```python
from build123d import *

# Parameters (mm, degrees)
SKETCH_1_W           = 80
SKETCH_1_H           = 60
SKETCH_1_R           = 2.1
SKETCH_1_W_2         = 40
SKETCH_1_H_2         = 24
EXTRUDE_1_DEPTH      = 10
CUT_EXTRUDE_1_DEPTH  = 80
SKETCH_5_W           = 5
SKETCH_5_H           = 3
CUT_EXTRUDE_2_DEPTH  = 80
SKETCH_7_W           = 56
SKETCH_7_H           = 24
CUT_EXTRUDE_3_DEPTH  = 1
SKETCH_8_W           = 40
SKETCH_8_H           = 40
EXTRUDE_2_DEPTH      = 3
SKETCH_9_W           = 10
SKETCH_9_H           = 60
CUT_EXTRUDE_4_DEPTH  = 10
CUT_EXTRUDE_11_DEPTH = 28
CUT_EXTRUDE_12_DEPTH = 41
SKETCH_24_W          = 10
SKETCH_24_H          = 10
EXTRUDE_3_DEPTH      = 70
SKETCH_25_W          = 12
SKETCH_25_H          = 6
CUT_EXTRUDE_13_DEPTH = 9
SKETCH_26_R          = 2
CUT_EXTRUDE_14_DEPTH = 8
CUT_EXTRUDE_15_REACH = 65.828
EXTRUDE_START        = -28
SKETCH_28_W          = 70
SKETCH_28_H          = 2
EXTRUDE_4_DEPTH      = 28
CUT_EXTRUDE_START    = -70
SKETCH_29_W          = 14
SKETCH_29_H          = 2
CUT_EXTRUDE_16_DEPTH = 70


with BuildPart() as part:
    # 草圖1 → 填料-伸長1 (new body)
    with BuildSketch(Plane(origin=(0, 0, 0), x_dir=(1, 0, 0), z_dir=(0, 1, 0))):
        Rectangle(SKETCH_1_W, SKETCH_1_H)
        with Locations(Location((-34.5, -5, 0), (0, 0, 270))):
            Circle(SKETCH_1_R, mode=Mode.SUBTRACT)
        with Locations(Location((-34.5, 5, 0), (0, 0, 270))):
            Circle(SKETCH_1_R, mode=Mode.SUBTRACT)
        with Locations(Location((15, -5, 0), (0, 0, 270))):
            Circle(SKETCH_1_R, mode=Mode.SUBTRACT)
        with Locations(Location((15, 5, 0), (0, 0, 270))):
            Circle(SKETCH_1_R, mode=Mode.SUBTRACT)
        with Locations((-10, 0)):
            Rectangle(SKETCH_1_W_2, SKETCH_1_H_2, mode=Mode.SUBTRACT)
    extrude(amount=EXTRUDE_1_DEPTH)

    # 草圖4 → 除料-伸長1 (cut)
    with BuildSketch(Plane(origin=(40, 0, 0), x_dir=(0, 0, -1), z_dir=(1, 0, 0))):
        Polygon((17, 10), (17, 8), (15, 8), (15, 3), (25, 3), (25, 8), (23, 8), (23, 10), align=None)
    extrude(amount=-CUT_EXTRUDE_1_DEPTH, mode=Mode.SUBTRACT)

    # 草圖5 → 除料-伸長2 (cut)
    with BuildSketch(Plane(origin=(0, 10, 0), x_dir=(1, 0, 0), z_dir=(0, 1, 0))):
        with Locations((12.5, 0)):
            Rectangle(SKETCH_5_W, SKETCH_5_H)
        with Locations((-32.5, 0)):
            Rectangle(SKETCH_5_W, SKETCH_5_H)
    extrude(amount=-CUT_EXTRUDE_2_DEPTH, mode=Mode.SUBTRACT)

    # 草圖7 → 除料-伸長3 (cut)
    with BuildSketch(Plane(origin=(0, 10, 0), x_dir=(1, 0, 0), z_dir=(0, 1, 0))):
        with Locations((-9.7, 0)):
            Rectangle(SKETCH_7_W, SKETCH_7_H)
    extrude(amount=-CUT_EXTRUDE_3_DEPTH, mode=Mode.SUBTRACT)

    # 草圖8 → 填料-伸長2 (add)
    with BuildSketch(Plane.ZY.offset(40)):
        with Locations((10, 5)):
            Rectangle(SKETCH_8_W, SKETCH_8_H)
    extrude(amount=EXTRUDE_2_DEPTH)

    # 草圖9 → 除料-伸長4 (cut)
    with BuildSketch(Plane(origin=(0, 10, 0), x_dir=(1, 0, 0), z_dir=(0, 1, 0))):
        with Locations((35, 0)):
            Rectangle(SKETCH_9_W, SKETCH_9_H)
    extrude(amount=-CUT_EXTRUDE_4_DEPTH, mode=Mode.SUBTRACT)

    # 草圖22 → 除料-伸長11 (cut)
    with BuildSketch(Plane(origin=(0, 10, 0), x_dir=(1, 0, 0), z_dir=(0, 1, 0))):
        Polygon((-43, -25), (-43, -30), (-38, -30), align=None)
    extrude(amount=-CUT_EXTRUDE_11_DEPTH, mode=Mode.SUBTRACT)

    # 草圖23 → 除料-伸長12 (cut)
    with BuildSketch(Plane(origin=(0, 25, 0), x_dir=(1, 0, 0), z_dir=(0, 1, 0))):
        Polygon((-43, -30), (-38, -30), (-43, -25), align=None)
    extrude(amount=-CUT_EXTRUDE_12_DEPTH, mode=Mode.SUBTRACT)

    # 草圖24 → 填料-伸長3 (add)
    with BuildSketch(Plane.ZY.offset(40)):
        with Locations((-35, 5)):
            Rectangle(SKETCH_24_W, SKETCH_24_H)
    extrude(amount=-EXTRUDE_3_DEPTH)

    # 草圖25 → 除料-伸長13 (cut)
    with BuildSketch(Plane(origin=(0, 10, 0), x_dir=(1, 0, 0), z_dir=(0, 1, 0))):
        with Locations((-12, 32)):
            Rectangle(SKETCH_25_W, SKETCH_25_H)
        with Locations((20, 32)):
            Rectangle(SKETCH_25_W, SKETCH_25_H)
    extrude(amount=-CUT_EXTRUDE_13_DEPTH, mode=Mode.SUBTRACT)

    # 草圖26 → 除料-伸長14 (cut)
    with BuildSketch(Plane(origin=(0, 0, -40), x_dir=(-1, 0, 0), z_dir=(0, 0, -1))):
        with Locations((-20, 4.723394197)):
            Circle(SKETCH_26_R)
        with Locations((12, 4.723394197)):
            Circle(SKETCH_26_R)
    extrude(amount=-CUT_EXTRUDE_14_DEPTH, mode=Mode.SUBTRACT)

    # 草圖27 → 除料-伸長15 (cut, up to next)
    with BuildSketch(Plane(origin=(0, 10, 0), x_dir=(1, 0, 0), z_dir=(0, 1, 0)), mode=Mode.PRIVATE) as cut_extrude_15_sk1:
        Polygon((30, -10), (20, -30), (30, -30), align=None)
    cut_extrude_15_tool1 = extrude(cut_extrude_15_sk1.sketch, amount=-CUT_EXTRUDE_15_REACH, mode=Mode.PRIVATE) & part.part
    add(cut_extrude_15_tool1.solids().sort_by_distance((26.666667, 10, 23.333333))[0], mode=Mode.SUBTRACT)

    # 草圖28 → 填料-伸長4 (add)
    with BuildSketch(Plane(origin=(0, 0, -40), x_dir=(-1, 0, 0), z_dir=(0, 0, -1)).offset(EXTRUDE_START)):
        with Locations((5, -1)):
            Rectangle(SKETCH_28_W, SKETCH_28_H)
    extrude(amount=EXTRUDE_4_DEPTH)

    # 草圖29 → 除料-伸長16 (cut)
    with BuildSketch(Plane(origin=(30, 0, 0), x_dir=(0, 0, -1), z_dir=(1, 0, 0)).offset(CUT_EXTRUDE_START)):
        with Locations((33, -1)):
            Rectangle(SKETCH_29_W, SKETCH_29_H)
    extrude(amount=CUT_EXTRUDE_16_DEPTH, mode=Mode.SUBTRACT)


solid = part.part
```
CAD build for the part. Positions are in the model's coordinates, mm. A direction names the side the tool comes from. Give positions to 0.01 mm unless a question says otherwise; leave off trailing zeros. Write each loop counter-clockwise with the first axis right and the second up, starting at its lowest first coordinate (ties: lowest second). Pieces come first, ordered by that corner, then holes. Notation, with made-up numbers: M 42.25,-39 L 68.25,-39 A11 cw 68.25,-34 Z; hole C 15,70.25 d6. An arc over 180 degrees is marked long. Return JSON: item names as keys, results as strings. Group by question number.
(1) Band-saw the part on C-C (x = -19.5). Give the cut face in (y, z), and give its area (3 significant figures).
(2) Mould opens along Z. For faces 1 (the face through (25, 5, 20)), 2 (the face through (21, 7, -35)), 3 (the face through (-5, -2, -19)), 4 (the face through (-5, -1, -26)) say: pulls with the +Z half, pulls with the -Z half, needs draft (parallel to the pull), parting line crosses it, or undercut.
(3) Drill centre lines: L1, parallel to Z at x = -34.5, y = 5.75; L2, parallel to Z at x = -10.5, y = 6; L3, parallel to Z at x = 5.5, y = 2.5. Where is each one in solid material? Low to high. Write a range as [from, to].
(4) Band-saw the part on A-A (x = -12). Give the cut face in (y, z).
(5) 3-axis set-ups, long thin cutter, end or side, ignore diameter. For faces 5 (the face through (-40, 2.6, -24.8)), 6 (the face through (20, 1, -32)), 7 (the face through (-10.53, 6.08, -37.53)), 8 (the face through (-5, 6, -15)), 9 (the face through (-33, 5, 1.5)): which of +Z, -Z, +X, -X, +Y, -Y reach the whole face in a straight line?
(6) Band-saw the part on D-D (z = 19). Give the cut face in (x, y).
(7) Band-saw the part on B-B (z = 5). Give the cut face in (x, y).
(8) Flat gauge pins, fed straight in: pin 1 Ø4 at (y, z) = (18, 1.5) entering from +X; pin 2 Ø7 at (x, z) = (6.5, -22) entering from -Y; pin 3 Ø3 at (x, z) = (-14, -28) entering from -Y. Where does each tip first touch, or does it go through?
Entries:
{
 "1": {"outline": "M -2,-26 L 0,-26 L 0,-40 L 10,-40 L 10,-23 L 8,-23 L 8,-25 L 3,-25 L 3,-15 L 8,-15 L 8,-17 L 10,-17 L 10,-12 L -2,-12 Z; M 0,12 L 10,12 L 10,30 L 0,30 Z", "area": "426 mm^2"},
 "2": {"face 1": "pulls with the +Z half", "face 2": "undercut", "face 3": "needs draft", "face 4": "pulls with the -Z half"},
 "3": {"L1": "z = [-40, -25], [-15, -7.1], [-2.9, -1.5], [1.5, 2.9], [7.1, 30]", "L2": "z = [-29, -25], [-15, -12], [12, 30]", "L3": "z = [-40, -12], [12, 30]"},
 "4": {"outline": "M -2,-26 L 0,-26 L 0,-40 L 2.72,-40 L 2.72,-35 L 1,-35 L 1,-29 L 10,-29 L 10,-23 L 8,-23 L 8,-25 L 3,-25 L 3,-15 L 8,-15 L 8,-17 L 10,-17 L 10,-12 L -2,-12 Z; M 0,12 L 10,12 L 10,30 L 0,30 Z; M 6.72,-40 L 10,-40 L 10,-35 L 6.72,-35 Z"},
 "5": {"face 5": "-Z, -X, +Y, -Y", "face 6": "+Y", "face 7": "-Z", "face 8": "+X, -X", "face 9": "+Y, -Y"},
 "6": {"outline": "M -43,-15 L -40,-15 L -40,0 L 25.5,0 L 25.5,10 L -40,10 L -40,25 L -43,25 Z"},
 "7": {"outline": "M -43,-15 L -40,-15 L -40,0 L -36.6,0 L -36.6,9 L -37.7,9 L -37.7,10 L -40,10 L -40,25 L -43,25 Z; M -32.4,0 L -30,0 L -30,9 L -32.4,9 Z; M 10,0 L 12.9,0 L 12.9,9 L 10,9 Z; M 17.1,0 L 30,0 L 30,10 L 18.3,10 L 18.3,9 L 17.1,9 Z"},
 "8": {"pin 1": "stops at x = -40", "pin 2": "stops at y = -2", "pin 3": "stops at y = 0"}
}
